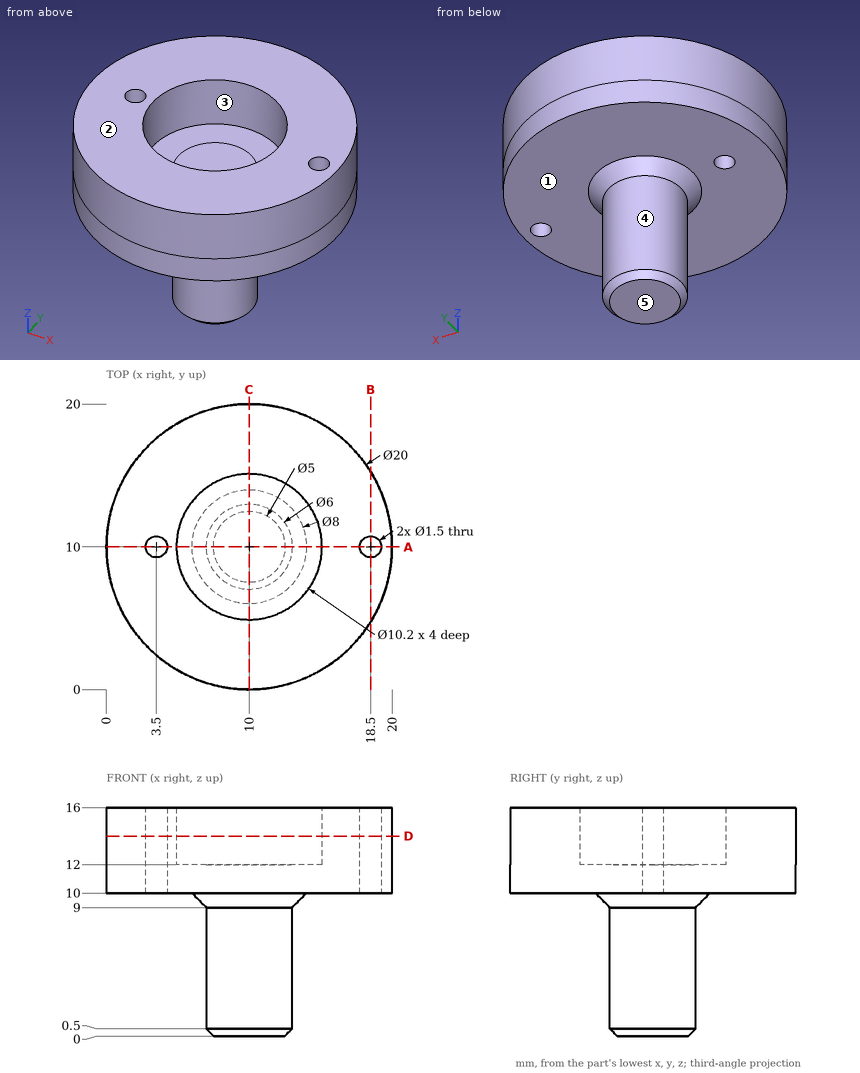
Answer from the drawing. Dimensions are ordinates in mm from the lowest x, y and z of the part. A direction names the side the tool comes from. Coordinates: 2 decimals unless noted, no trailing zeros. Loops run counter-clockwise (first coordinate to the right, second up) from the corner with the lowest first, then second, coordinate; pieces in that order, holes last. Notation, with made-up numbers: (-21, 73) -> (34, 73) arc R18 ccw to (34, 106) -> close; hole circle Ø2 at (-2, -12.75). An arc over 180 degrees is marked (long way). Answer in a Markdown table with one row per item.
Item 1: For a pull along X with two mould halves and no side action, classify the marked faces 3, 4 and 5 as released by +X, released by -X, zero draft, split by the parting line, or undercut.
Returned:
| item | result |
|---|---|
| face 3 | undercut |
| face 4 | split by the parting line |
| face 5 | zero draft |
Item 2: A cutting plane is placed at A-A on y = 10. Determine the outline of the cut face in (x, z), plus the area to 3 significant figures.
Returned:
| item | result |
|---|---|
| outline | (0, 10) -> (2.75, 10) -> (2.75, 16) -> (0, 16) -> close; (4.25, 10) -> (6, 10) -> (7, 9) -> (7, 0.5) -> (7.5, 0) -> (12.5, 0) -> (13, 0.5) -> (13, 9) -> (14, 10) -> (17.75, 10) -> (17.75, 16) -> (15.1, 16) -> (15.1, 12) -> (4.9, 12) -> (4.9, 16) -> (4.25, 16) -> close; (19.25, 10) -> (20, 10) -> (20, 16) -> (19.25, 16) -> close |
| area | 122 mm^2 |
Item 3: Straight lines are drawn through the part: line 1 along Y through (x, z) = (10, 14.6); line 2 along Z through (x, y) = (16, 12); line 3 along Y through (x, z) = (18.5, 11.7). For each, find the intervals that lie inside material, in ascending order. Write a range as [from, to].
Returned:
| item | result |
|---|---|
| line 1 | y = [0, 4.9], [15.1, 20] |
| line 2 | z = [10, 16] |
| line 3 | y = [4.73, 9.25], [10.75, 15.27] |
Item 4: A cutting plane is placed at B-B on x = 18.5. Determine the outline of the cut face in (y, z), plus the area to 3 significant figures.
Returned:
| item | result |
|---|---|
| outline | (4.73, 10) -> (9.25, 10) -> (9.25, 16) -> (4.73, 16) -> close; (10.75, 10) -> (15.27, 10) -> (15.27, 16) -> (10.75, 16) -> close |
| area | 54.2 mm^2 |
Item 5: A cutting plane is placed at D-D on z = 14. Determine the outline of the cut face in (x, y).
Returned:
| item | result |
|---|---|
| outline | circle Ø20 at (10, 10); hole circle Ø1.5 at (3.5, 10); hole circle Ø10.2 at (10, 10); hole circle Ø1.5 at (18.5, 10) |
Item 6: Each of these flat-tipped pins is pushed along its axis until it touches: P1, Ø2, axis at x = 6.5, z = 13.5, coming from the +Y side; P2, Ø5, axis at x = 8.5, y = 8.5, coming from the +Z side; P3, Ø6, axis at y = 6.5, z = 7.5, coming from the -X side. Where does it stop, or does it pass through?
Returned:
| item | result |
|---|---|
| P1 | stops at y = 19.68 |
| P2 | stops at z = 12 |
| P3 | stops at x = 0.17 |
Item 7: A cutting plane is placed at C-C on x = 10. Determine the outline of the cut face in (y, z), plus the area to 3 significant figures.
Returned:
| item | result |
|---|---|
| outline | (0, 10) -> (6, 10) -> (7, 9) -> (7, 0.5) -> (7.5, 0) -> (12.5, 0) -> (13, 0.5) -> (13, 9) -> (14, 10) -> (20, 10) -> (20, 16) -> (15.1, 16) -> (15.1, 12) -> (4.9, 12) -> (4.9, 16) -> (0, 16) -> close |
| area | 140 mm^2 |
Item 8: For the marked faces 1 and 2, determine the directions among +Z, -Z, +X, -X, +Y, -Y from which every point of the face is accessible in a straight line to the end or side of a thin tool.
Returned:
| item | result |
|---|---|
| face 1 | -Z |
| face 2 | +Z, +X, -X, +Y, -Y |
